```python
from build123d import *

# Parameters (mm, degrees)
SKETCH_1_W          = 10
SKETCH_1_H          = 10
EXTRUDE_1_DEPTH     = 2
SKETCH_2_W          = 10
SKETCH_2_H          = 12
EXTRUDE_2_DEPTH     = 2
EXTRUDE_4_DEPTH     = 2
EXTRUDE_START       = -2
EXTRUDE_5_DEPTH     = 2
SKETCH_5_R          = 1
CUT_EXTRUDE_1_DEPTH = 10


with BuildPart() as part:
    # 草图1 → 凸台-拉伸1 (new body)
    with BuildSketch(Plane.XY):
        with Locations((5, 5)):
            Rectangle(SKETCH_1_W, SKETCH_1_H)
    extrude(amount=EXTRUDE_1_DEPTH)

    # 草图2 → 凸台-拉伸2 (add)
    with BuildSketch(Plane.XZ):
        with Locations((5, 6)):
            Rectangle(SKETCH_2_W, SKETCH_2_H)
    extrude(amount=EXTRUDE_2_DEPTH)

    # 草图3 → 凸台-拉伸4 (add)
    with BuildSketch(Plane(origin=(10, 0, 0), x_dir=(0, 0, -1), z_dir=(1, 0, 0))):
        with BuildLine():
            Line((0, -2), (-12, -2))
            Line((-12, -2), (0.083847107, -7.738286318))
            ThreePointArc((0.083847107, -7.738286318), (5.656854249, -7.656854249), (5.738286318, -2.083847107))
            Line((5.738286318, -2.083847107), (0, 10))
            Line((0, 10), (0, -2))
        make_face()
    extrude(amount=-EXTRUDE_4_DEPTH)

    # 草图4 → 凸台-拉伸5 (add)
    with BuildSketch(Plane.ZY.offset(EXTRUDE_START)):
        with BuildLine():
            Line((0, -2), (0, 10))
            Line((0, 10), (-5.738286318, -2.083847107))
            ThreePointArc((-5.738286318, -2.083847107), (-5.656854249, -7.656854249), (-0.083847107, -7.738286318))
            Line((-0.083847107, -7.738286318), (12, -2))
            Line((12, -2), (0, -2))
        make_face()
    extrude(amount=EXTRUDE_5_DEPTH)

    # 草图5 → 切除-拉伸1 (cut)
    with BuildSketch(Plane(origin=(10, 0, 0), x_dir=(0, 0, -1), z_dir=(1, 0, 0))):
        with Locations((2.828427125, -4.828427125)):
            Circle(SKETCH_5_R)
    extrude(amount=-CUT_EXTRUDE_1_DEPTH, mode=Mode.SUBTRACT)


solid = part.part
```
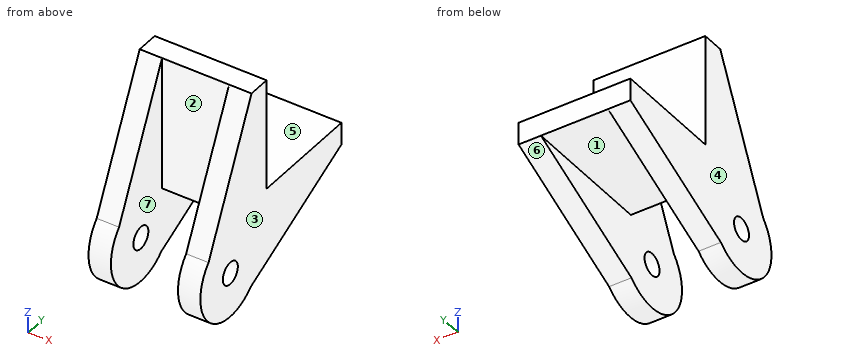
Source: CAD feature listing. Evaluate the final solid. Frame: model axes, mm. Face numbers are marked on the shaded views. A direction names the side the tool comes from. Round coordinates to 2 decimals unless told otherwise and drop trailing zeros. Loops run counter-clockwise (first coordinate to the right, second up) from the corner with the lowest first, then second, coordinate; pieces in that order, holes last. Notation, with made-up numbers: M 63.5,-3.75 L 112.5,-3.75 A14 cw 112.5,16.25 Z; hole C 62.25,36.5 d11. An arc over 180 degrees is marked long. Use a Markdown table: item, result. Add a question column.
1. Contact query for flat-ended pins moving along their axis: pin 1 (1.5 mm diameter, centred on x = 5, y = 0, fed in from -Z); pin 2 (1.8 mm diameter, centred on x = 5.5, z = 9, fed in from -Y); pin 3 (5 mm diameter, centred on x = 4.5, z = 8, fed in from +Y). Output: stop coordinate, or through.
2. Cut plane B-B, the plane z = 3.5. Output: boundary loops of the cut face in (x, y).
3. Cut plane C-C, the plane y = 5.75. Output: boundary loops of the cut face in (x, z), and give its area (3 significant figures).
4. Pull-direction query (X, two-part tool) for the marked faces 1, 2, 3 and 4; classes: +X half, -X half, draft (parallel to the pull), parting line (faces both ways), or undercut.
5. Set-up query: the marked faces 5, 6 and 7. Return all of +Z, -Z, +X, -X, +Y, -Y with unobstructed straight access to the full face (end or side cutting, diameter ignored); none if empty.
6. Cut plane A-A, the plane y = -7.25. Output: boundary loops of the cut face in (x, z), and give its area (3 significant figures).
7. Cut plane D-D, the plane x = 2.5. Output: boundary loops of the cut face in (y, z), and give its area (3 significant figures).
8. Ray query, line 1 along X through (y, z) = (-2.25, -5.5); line 2 along Y through (x, z) = (5.75, 4.25); line 3 along Z through (x, y) = (5, 2). Return the intervals inside material, ascending. Write a range as [from, to].
Solution:
| question | item | result |
|---|---|---|
| 1 | pin 1 | stops at z = 0 |
| 1 | pin 2 | stops at y = -2 |
| 1 | pin 3 | stops at y = 0 |
| 2 | outline | M 0,-6.04 L 2,-6.04 L 2,-2 L 8,-2 L 8,-6.04 L 10,-6.04 L 10,0 L 0,0 Z |
| 3 | outline | M 0,-2.02 L 2,-2.02 L 2,0 L 8,0 L 8,-2.02 L 10,-2.02 L 10,2 L 0,2 Z |
| 3 | area | 28.1 mm2 |
| 4 | face 1 | undercut |
| 4 | face 2 | undercut |
| 4 | face 3 | +X half |
| 4 | face 4 | -X half |
| 5 | face 5 | +Z, +X, -X, +Y |
| 5 | face 6 | -Z, +X, -X, +Y |
| 5 | face 7 | -Z, -Y |
| 6 | outline | M 0,-6.01 L 2,-6.01 L 2,0.94 L 0,0.94 Z; M 8,-6.01 L 10,-6.01 L 10,0.94 L 8,0.94 Z |
| 6 | area | 27.8 mm2 |
| 7 | outline | M -2,0 L 10,0 L 10,2 L 0,2 L 0,12 L -2,12 Z |
| 7 | area | 44.0 mm2 |
| 8 | line 1 | x = [0, 2], [8, 10] |
| 8 | line 2 | y = [-2, 0] |
| 8 | line 3 | z = [0, 2] |
